```python
from build123d import *

# Parameters (mm, degrees)
SKETCH1_W               = 53.975
SKETCH1_H               = 38.1
BOSS_EXTRUDE1_DEPTH     = 2.38125
CHAMFER1_SIZE           = 3.175
CUT_EXTRUDE1_DEPTH      = 34.375276216
CUT_EXTRUDE1_DEPTH_BACK = 34.375276216
SKETCH4_W               = 28.575
SKETCH4_H               = 28.575
FILLET1_R               = 6.35


with BuildPart() as part:
    # Sketch1 → Boss-Extrude1 (new, symmetric)
    with BuildSketch(Plane(origin=(0, 0, 0), x_dir=(1, 0, 0), z_dir=(0, 1, 0))):
        Rectangle(SKETCH1_W, SKETCH1_H)
    extrude(amount=BOSS_EXTRUDE1_DEPTH, both=True)

    # Chamfer1
    chamfer1_edges = [part.edges().sort_by_distance(p)[0] for p in [
        (26.9875, 2.38125, 0),
    ]]
    chamfer(chamfer1_edges, length=CHAMFER1_SIZE)

    # Sketch4 → Cut-Extrude1 (cut, two sides: drawn at the far end of the back side and taken through both)
    with BuildSketch(Plane(origin=(0, 2.38125, 0), x_dir=(1, 0, 0), z_dir=(0, 1, 0)).offset(-CUT_EXTRUDE1_DEPTH_BACK)):
        Rectangle(SKETCH4_W, SKETCH4_H)
    extrude(amount=CUT_EXTRUDE1_DEPTH + CUT_EXTRUDE1_DEPTH_BACK, mode=Mode.SUBTRACT)

    # Fillet1
    fillet1_edges = [part.edges().sort_by_distance(p)[0] for p in [
        (-14.2875, 0, 14.2875),
        (-14.2875, 0, -14.2875),
        (14.2875, 0, -14.2875),
        (14.2875, 0, 14.2875),
    ]]
    fillet(fillet1_edges, radius=FILLET1_R)


solid = part.part
```
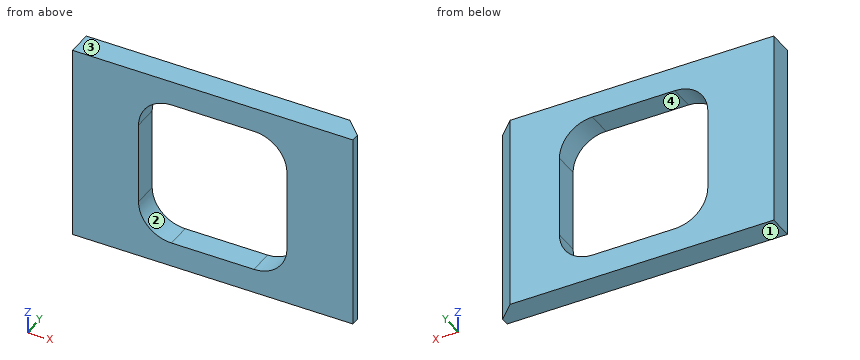
Part model, mm, in its own coordinate system. Face numbers are marked on the shaded views. A direction names the side the tool comes from. Give positions to 0.01 mm unless a question says otherwise; leave off trailing zeros. Loops run counter-clockwise (first coordinate to the right, second up) from the corner with the lowest first, then second, coordinate; pieces in that order, holes last. Notation, with made-up numbers: M -17,58 L 13,58 A7 ccw 13,70 Z; hole C 47,26.25 d5. An arc over 180 degrees is marked long. Return JSON: item names as keys, results as strings.
1) Pull direction X, two halves, no side cores. Call the marked faces 1 and 2: released by +X, released by -X, zero draft, split by the parting line, or undercut.
Calculated:
{"face 1": "zero draft", "face 2": "undercut"}
2) Saw through at D-D, the plane y = 0.55. List the corners of the cut face in (x, z).
Calculated:
{"outline": "M -26.99,-19.05 L 25.64,-19.05 L 25.64,19.05 L -26.99,19.05 Z; hole M -14.29,-7.94 A6.35 ccw -7.94,-14.29 L 7.94,-14.29 A6.35 ccw 14.29,-7.94 L 14.29,7.94 A6.35 ccw 7.94,14.29 L -7.94,14.29 A6.35 ccw -14.29,7.94 Z"}
3) Saw through at B-B, the plane z = -7. List the corners of the cut face in (x, y).
Calculated:
{"outline": "M -26.99,-2.38 L -14.29,-2.38 L -14.29,2.38 L -26.99,2.38 Z; M 14.29,-2.38 L 26.99,-2.38 L 26.99,-0.79 L 23.81,2.38 L 14.29,2.38 Z"}
4) Saw through at C-C, the plane z = 15. List the corners of the cut face in (x, y), then the cut area to 3 significant figures.
Calculated:
{"outline": "M -26.99,-2.38 L 26.99,-2.38 L 26.99,-0.79 L 23.81,2.38 L -26.99,2.38 Z", "area": "252 mm2"}
5) Saw through at A-A, the plane x = 5.5. List the corners of the cut face in (y, z).
Calculated:
{"outline": "M -2.38,-19.05 L 2.38,-19.05 L 2.38,-14.29 L -2.38,-14.29 Z; M -2.38,14.29 L 2.38,14.29 L 2.38,19.05 L -2.38,19.05 Z"}
6) Flat gauge pins, fed straight in: pin 1 Ø12 at (x, z) = (2, -3.5) entering from +Y; pin 2 Ø2.5 at (y, z) = (0, 0) entering from +X. Where does each tip first touch, or does it go through?
Calculated:
{"pin 1": "passes through", "pin 2": "stops at x = 26.99"}
7) Drill centre lines: line 1 (Z direction, x = -7.5, y = 1.7); line 2 (X direction, y = -1.55, z = -6.5); line 3 (X direction, y = 0.05, z = 0.5). Where is each one in solid material? Low to high.
Calculated:
{"line 1": "z = -19.05 to -14.29, 14.29 to 19.05", "line 2": "x = -26.99 to -14.29, 14.29 to 26.99", "line 3": "x = -26.99 to -14.29, 14.29 to 26.14"}
8) 3-axis set-ups, long thin cutter, end or side, ignore diameter. For the marked faces 3 and 4: which of +Z, -Z, +X, -X, +Y, -Y reach the whole face in a straight line?
Calculated:
{"face 3": "+Z, +X, -X, +Y, -Y", "face 4": "+Y, -Y"}
